Autodesk Inventor part; units mm, degrees
ref_plane "YZ Plane" through (0, 0, 0) normal (1, 0, 0) x (0, 1, 0)
ref_plane "XZ Plane" through (0, 0, 0) normal (0, 1, 0) x (-1, 0, 0)
ref_plane "XY Plane" through (0, 0, 0) normal (0, 0, 1) x (1, 0, 0)
sketch "Sketch1" plane through (0, 0, 0) normal (0, 0, 1) x (1, 0, 0)
  line L0 (0, 120) -> (-30, 120)
  line L1 (-30, 120) -> (-30, 80)
  line L2 (-30, 80) -> (0, 80)
  line L3 (-20, 110) -> (-10, 110)
  line L4 (-10, 110) -> (-10, 90)
  line L5 (-10, 90) -> (-20, 90)
  line L6 (-20, 90) -> (-20, 110)
  line L7 (0, 120) -> (3, 120)
  line L8 (3, 120) -> (3, 80)
  line L9 (3, 80) -> (0, 80)
  line L10 (-30, 120) -> (3, 120)
  line L11 (3, 120) -> (3, 80)
  line L12 (3, 80) -> (-30, 80)
  line L13 (-30, 80) -> (-30, 120)
  point P0 (0, 0)
extrude "Extrusion1" add sketch "Sketch1" along normal blind 3
properties part number "kunci"
Design review of the part built by this model. Coordinates are the model's own, in mm. A direction names the side the tool comes from. Give positions to 0.01 mm unless a question says otherwise; leave off trailing zeros. Order: outer loops, then holes, each group sorted by start corner. A loop starts at its lowest first (then second) coordinate and runs counter-clockwise, first axis right, second up. Notation, with made-up numbers: (-12, 82) - (29, 82) arc R19 ccw to (29, 105) - close; hole circle Ø6 at (-4, 30.25). An arc over 180 degrees is marked (long way). Use a Markdown table: item, result. Add a question column.
(1) Add section A-A on x = -18. Give the boundary of the cut face in (y, z).
(2) Wall thickness on probe 1 along Y at (x, z) = (-19, 1.9); probe 2 along X at (y, z) = (102.5, 2.05): over which ranges is each line inside the solid? List them lowest first. Write a range as [from, to].
(3) Clearance check with a flat-ended pin moving along its axis: P1, Ø8, axis at x = -26.5, y = 86.5, coming from the -Z side. State where the tip first meets the part, or that it passes through.
(4) Machinability: for faces 4 (the face through (-30, 100, 1)), 5 (the face through (-20, 100, 1)), which of the approach directions +Z, -Z, +X, -X, +Y, -Y give a long, thin tool a straight path to every point of the face, cutting with its end or side? Answer none if there is none.
(5) Mouldability with a two-part tool opening along Y and no side actions: class faces 1 (the face through (-21, 100, 3)), 2 (the face through (-15, 90, 1)), 3 (the face through (-14, 120, 1)) as +Y half, -Y half, draft (parallel to the pull), parting line (faces both ways), or undercut.
(6) Add section B-B on z = 2.5. Give the boundary of the cut face in (x, y).
(7) Add section C-C on y = 109. Give the boundary of the cut face in (x, z).
Report:
| question | item | result |
|---|---|---|
| 1 | outline | (80, 0) - (90, 0) - (90, 3) - (80, 3) - close; (110, 0) - (120, 0) - (120, 3) - (110, 3) - close |
| 2 | probe 1 | y = [80, 90], [110, 120] |
| 2 | probe 2 | x = [-30, -20], [-10, 3] |
| 3 | P1 | stops at z = 0 |
| 4 | face 4 | +Z, -Z, -X, +Y, -Y |
| 4 | face 5 | +Z, -Z |
| 5 | face 1 | draft |
| 5 | face 2 | undercut |
| 5 | face 3 | +Y half |
| 6 | outline | (-30, 80) - (3, 80) - (3, 120) - (-30, 120) - close; hole (-20, 90) - (-10, 90) - (-10, 110) - (-20, 110) - close |
| 7 | outline | (-30, 0) - (-20, 0) - (-20, 3) - (-30, 3) - close; (-10, 0) - (3, 0) - (3, 3) - (-10, 3) - close |
